Source: CAD feature listing. Evaluate the final solid. Frame: model axes, mm. A direction names the side the tool comes from. Give positions to 0.01 mm unless a question says otherwise; leave off trailing zeros. Loops run counter-clockwise (first coordinate to the right, second up) from the corner with the lowest first, then second, coordinate; pieces in that order, holes last. Notation, with made-up numbers: (-35.5, 57.25) - (-5.5, 57.25) arc R9 cw to (-5.5, 62.25) - close; hole circle Ø8 at (-21, 66). An arc over 180 degrees is marked (long way). Put each result on its own line as item: value.
```python
from build123d import *

# Parameters (mm, degrees)
SKETCH1_W                       = 135
SKETCH1_H                       = 80
SKETCH1_R                       = 15
BOSS_EXTRUDE1_DEPTH             = 8
CBORE_FOR_M2_5_SHCS1_AT_2_COUNT = 2
CBORE_FOR_M2_5_SHCS1_AT_2_PITCH = 52
CBORE_FOR_M2_5_SHCS1_AT_3_COUNT = 2
CBORE_FOR_M2_5_SHCS1_AT_3_PITCH = 58.591808301
CBORE_FOR_M2_5_SHCS1_AT_4_COUNT = 2
CBORE_FOR_M2_5_SHCS1_AT_4_PITCH = 27
M5_CLEARANCE_HOLE1_D            = 5.3
M5_CLEARANCE_HOLE1_CSINK_D      = 5.35
M5_CLEARANCE_HOLE1_CSINK_ANGLE  = 90
CBORE_FOR_M4_SHCS1_AT_2_COUNT   = 2
CBORE_FOR_M4_SHCS1_AT_2_PITCH   = 60
CBORE_FOR_M4_SHCS1_AT_3_COUNT   = 2
CBORE_FOR_M4_SHCS1_AT_3_PITCH   = 120
CBORE_FOR_M4_SHCS1_AT_4_COUNT   = 2
CBORE_FOR_M4_SHCS1_AT_4_PITCH   = 64
CBORE_FOR_M4_SHCS1_AT_5_COUNT   = 2
CBORE_FOR_M4_SHCS1_AT_5_PITCH   = 87.726848798
FILLET1_R                       = 20


with BuildPart() as part:
    # Sketch1 → Boss-Extrude1 (new body)
    with BuildSketch(Plane.XY):
        with Locations((14, 10)):
            Rectangle(SKETCH1_W, SKETCH1_H)
        Circle(SKETCH1_R, mode=Mode.SUBTRACT)
    extrude(amount=BOSS_EXTRUDE1_DEPTH)

    # Sketch3 → CBORE for M2.5 SHCS1 (revolve, cut)
    with BuildSketch(Plane(origin=(10.5, 13.5, 8), x_dir=(0, -1, 0), z_dir=(1, 0, 0))):
        Polygon((0, 0), (0, 8), (1.45, 8), (1.45, 2.5), (2.75, 2.5), (2.75, 0.025), (2.775, 0), align=None)
    cbore_for_m2_5_shcs1 = revolve(axis=Axis((10.5, 13.5, 14.35), (0, 0, -1)), mode=Mode.SUBTRACT)

    # CBORE for M2.5 SHCS1 at 2: CBORE for M2.5 SHCS1 ×2
    with Locations(*[(-i * CBORE_FOR_M2_5_SHCS1_AT_2_PITCH, 0, 0) for i in range(1, CBORE_FOR_M2_5_SHCS1_AT_2_COUNT)]):
        add(cbore_for_m2_5_shcs1, mode=Mode.SUBTRACT)

    # CBORE for M2.5 SHCS1 at 3: CBORE for M2.5 SHCS1 ×2
    with Locations(*[Vector(-0.8874960768017396, -0.4608152706470573, 0) * (i * CBORE_FOR_M2_5_SHCS1_AT_3_PITCH) for i in range(1, CBORE_FOR_M2_5_SHCS1_AT_3_COUNT)]):
        add(cbore_for_m2_5_shcs1, mode=Mode.SUBTRACT)

    # CBORE for M2.5 SHCS1 at 4: CBORE for M2.5 SHCS1 ×2
    with Locations(*[(0, -i * CBORE_FOR_M2_5_SHCS1_AT_4_PITCH, 0) for i in range(1, CBORE_FOR_M2_5_SHCS1_AT_4_COUNT)]):
        add(cbore_for_m2_5_shcs1, mode=Mode.SUBTRACT)

    # Sketch4 → Cut-Revolve1 (revolve, cut)
    with BuildSketch(Plane(origin=(60, 0, 0), x_dir=(0, 0, -1), z_dir=(1, 0, 0)), mode=Mode.PRIVATE) as cut_revolve1_sk:
        Polygon((-8, 26), (0, 26), (0, 39.5), (-6, 39.5), (-6, 38.5), (-8, 38.5), align=None)
    revolve(cut_revolve1_sk.sketch.rotate(Axis((60, 26, 0), (0, 0, 1)), 90), axis=Axis((60, 26, 0), (0, 0, 1)), mode=Mode.SUBTRACT)

    # M5 Clearance Hole1 (through all)
    with Locations(Plane(origin=(0, 0, 0), x_dir=(-1, 0, 0), z_dir=(0, 0, -1))):
        with Locations((-16.057223443, 23.305912883), (-27.985446572, -4.220755876)):
            CounterSinkHole(M5_CLEARANCE_HOLE1_D / 2, M5_CLEARANCE_HOLE1_CSINK_D / 2, counter_sink_angle=M5_CLEARANCE_HOLE1_CSINK_ANGLE)

    # Sketch13 → CBORE for M4 SHCS1 (revolve, cut)
    with BuildSketch(Plane(origin=(-46, -22, 8), x_dir=(0, -1, 0), z_dir=(1, 0, 0))):
        Polygon((0, 0), (0, 8), (2.25, 8), (2.25, 4), (4, 4), (4, 0.025), (4.025, 0), align=None)
    cbore_for_m4_shcs1 = revolve(axis=Axis((-46, -22, 14.35), (0, 0, -1)), mode=Mode.SUBTRACT)

    # CBORE for M4 SHCS1 at 2: CBORE for M4 SHCS1 ×2
    with Locations(*[(i * CBORE_FOR_M4_SHCS1_AT_2_PITCH, 0, 0) for i in range(1, CBORE_FOR_M4_SHCS1_AT_2_COUNT)]):
        add(cbore_for_m4_shcs1, mode=Mode.SUBTRACT)

    # CBORE for M4 SHCS1 at 3: CBORE for M4 SHCS1 ×2
    with Locations(*[(i * CBORE_FOR_M4_SHCS1_AT_3_PITCH, 0, 0) for i in range(1, CBORE_FOR_M4_SHCS1_AT_3_COUNT)]):
        add(cbore_for_m4_shcs1, mode=Mode.SUBTRACT)

    # CBORE for M4 SHCS1 at 4: CBORE for M4 SHCS1 ×2
    with Locations(*[(0, i * CBORE_FOR_M4_SHCS1_AT_4_PITCH, 0) for i in range(1, CBORE_FOR_M4_SHCS1_AT_4_COUNT)]):
        add(cbore_for_m4_shcs1, mode=Mode.SUBTRACT)

    # CBORE for M4 SHCS1 at 5: CBORE for M4 SHCS1 ×2
    with Locations(*[Vector(0.6839411288813297, 0.7295372041400852, 0) * (i * CBORE_FOR_M4_SHCS1_AT_5_PITCH) for i in range(1, CBORE_FOR_M4_SHCS1_AT_5_COUNT)]):
        add(cbore_for_m4_shcs1, mode=Mode.SUBTRACT)

    # Fillet1
    fillet1_edges = [part.edges().sort_by_distance(p)[0] for p in [
        (81.5, 50, 4),
    ]]
    fillet(fillet1_edges, radius=FILLET1_R)


solid = part.part
```
1) Mould query, pull axis Y, two halves, no side actions, for faces 1 (the cylindrical face through (75.486, 44.297, 4.056)), 2 (the flat face through (-44, 44, 4)), 3 (the flat face through (13, 11, 8)). Classes: pulls with the +Y half, pulls with the -Y half, needs draft (parallel to the pull), parting line crosses it, or undercut.
Check result:
face 1: pulls with the +Y half
face 2: undercut
face 3: needs draft
2) Pin query (flat end, axial travel): P1, Ø1.7, axis at x = 10.5, y = -13.5, coming from the -Z side; P2, Ø1.6, axis at x = -43, y = -14.5, coming from the +Z side; P3, Ø7, axis at x = 14, y = 42, coming from the +Z side; P4, Ø5, axis at x = -18.5, y = 16.5, coming from the -Z side. Return the tip coordinate at first contact, or that it passes through.
Check result:
P1: through
P2: z = 5.5
P3: z = 4
P4: z = 0
3) Section query C-C, the plane y = -22. State how many separate pieces and enclosed holes the cut face has, plus the area to 3 significant figures.
Check result:
separate pieces: 4
enclosed holes: 0
area: 930 mm²
4) Access query for faces 4 (the cylindrical face through (-48.23, 42.29, 2.03)), 5 (the cylindrical face through (73.487, 25.406, 3.042)), 6 (the flat face through (-40, -12, 5.5)). Directions: +Z, -Z, +X, -X, +Y, -Y. A direction counts if a zero-diameter tool reaches every point of the face in a straight line with its end or side. Return the directions, or none.
Check result:
face 4: +Z, -Z
face 5: -Z
face 6: +Z
5) Section query A-A, the plane y = 0. Output: boundary loops of the cut face in (x, z).
Check result:
outline: (-53.5, 0) - (-15, 0) - (-15, 8) - (-53.5, 8) - close; (15, 0) - (81.5, 0) - (81.5, 8) - (15, 8) - close
6) Material intervals for line 1 along X through (y, z) = (-22, 6.4); line 2 along X through (y, z) = (-2.5, 4.25); line 3 along Y through (x, z) = (0, 5.5), sorted ascending. Write a range as [from, to].
Check result:
line 1: [-53.5, -50], [-42, 10], [18, 70], [78, 81.5]
line 2: [-53.5, -14.79], [14.79, 25.97], [30, 81.5]
line 3: [-30, -15], [15, 50]
7) Section query B-B, the plane x = -46. Output: boundary loops of the cut face in (y, z) (3 decimals), plus the area to 3 significant figures.
Check result:
outline: (-30, 0) - (-24.25, 0) - (-24.25, 4) - (-26, 4) - (-26, 7.975) - (-26.025, 8) - (-30, 8) - close; (-19.75, 0) - (39.75, 0) - (39.75, 4) - (38, 4) - (38, 7.975) - (37.975, 8) - (-17.975, 8) - (-18, 7.975) - (-18, 4) - (-19.75, 4) - close; (44.25, 0) - (50, 0) - (50, 8) - (46.025, 8) - (46, 7.975) - (46, 4) - (44.25, 4) - close
area: 540 mm²
